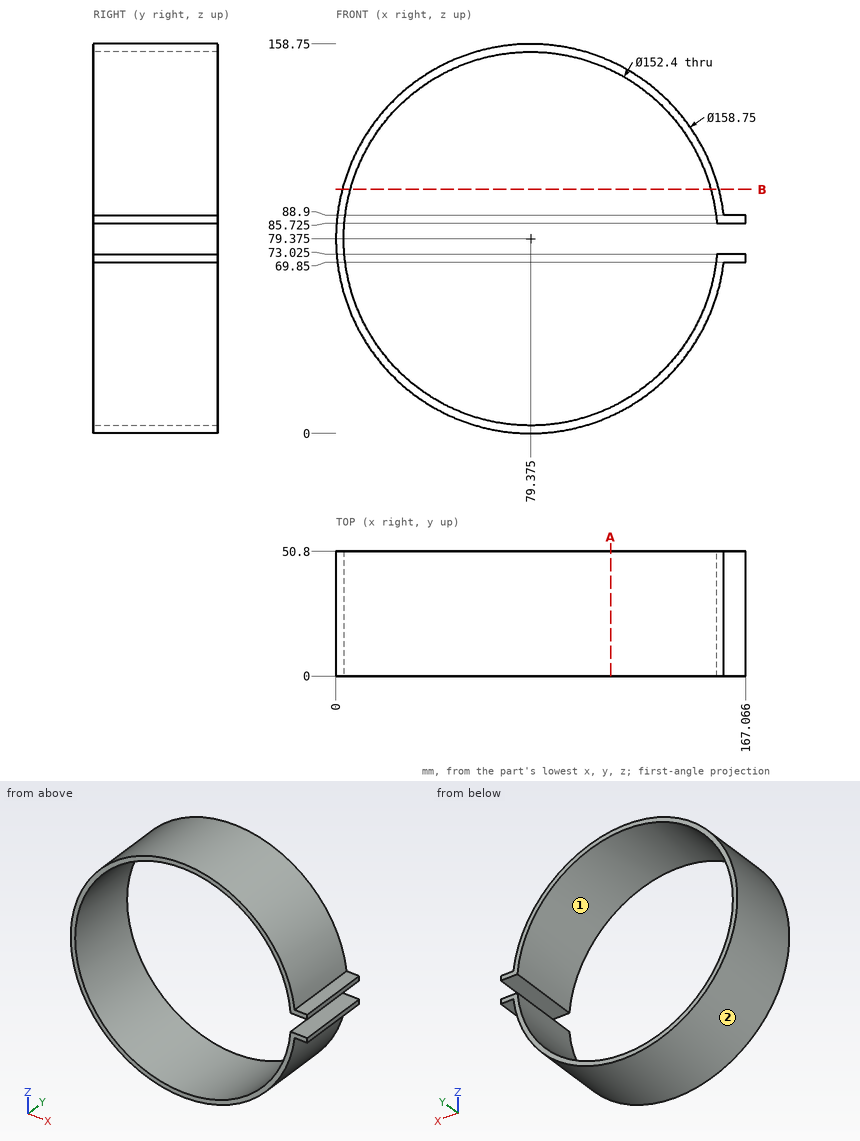
For this review, use the dimensioned drawing (mm, ordinates from the lowest corner) and the shaded views. Give positions to 0.01 mm unless a question says otherwise; leave off trailing zeros. Order: outer loops, then holes, each group sorted by start corner. A loop starts at its lowest first (then second) coordinate and runs counter-clockwise, first axis right, second up.
1) Wall thickness on line 1 (Z direction, x = 81.5, y = 42.5); line 2 (Z direction, x = 48.5, y = 43); line 3 (X direction, y = 45.5, z = 47): over which ranges is each line inside the solid? List them lowest first.
2) Insertion check: pin 1 (13 mm diameter, centred on x = 158.5, y = 36, fed in from +Z); pin 2 (1 mm diameter, centred on x = 23, y = 26.5, fed in from +Z); pin 3 (4.5 mm diameter, centred on x = 161.5, y = 16.5, fed in from -Z). Each pin has a flat end and moves straight along its axis. Give the tip position at first contact, or say it passes through.
3) Take a section at A-A (x = 112). Give the boundary of the cut face in (y, z).
4) Take a section at B-B (z = 99.5). Give the boundary of the cut face in (x, y), then the cut area to 3 significant figures.
5) The part is to be moulded in two halves that separate along X. For the marked faces 1 and 2, say which applies: released by +X, released by -X, zero draft, split by the parting line, or undercut.
Derived:
1. line 1: z = 0.03 to 3.2, 155.55 to 158.72
1. line 2: z = 6.25 to 9.71, 149.04 to 152.5
1. line 3: x = 6.9 to 10.39, 148.36 to 151.85
2. pin 1: stops at z = 111.41
2. pin 2: stops at z = 135.75
2. pin 3: stops at z = 69.85
3. outline: (0, 7.01) - (50.8, 7.01) - (50.8, 10.51) - (0, 10.51) - close; (0, 148.24) - (50.8, 148.24) - (50.8, 151.74) - (0, 151.74) - close
4. outline: (2.59, 0) - (5.88, 0) - (5.88, 50.8) - (2.59, 50.8) - close; (152.87, 0) - (156.16, 0) - (156.16, 50.8) - (152.87, 50.8) - close
4. area: 334 mm2
5. face 1: undercut
5. face 2: split by the parting line
